Autodesk Fusion 360 part; units mm, degrees
sketch "Sketch1" plane through (0, 0, 0) normal (0, 0, 1) x (1, 0, 0)
  circle A0 centre (0, 0) radius 3.45
  circle A1 centre (0, 0) radius 4.45
  dimension "d1" = 6.9
  dimension "d2" = 1
extrude "Extrude1" add sketch "Sketch1" along normal blind 3
extrude "Extrude2" add sketch "Sketch1" along normal blind 6 contours A0
sketch "Sketch2" plane through (0, 0, 6) normal (0, 0, 1) x (-1, 0, 0)
  circle A0 centre (0, 0) radius 3.45
  circle A1 centre (-2, 2) radius 0.5
  circle A2 centre (0, 2) radius 0.5
  circle A3 centre (2, 2) radius 0.5
  circle A4 centre (-2, 0) radius 0.5
  circle A5 centre (0, 0) radius 0.5
  circle A6 centre (2, 0) radius 0.5
  circle A7 centre (-2, -2) radius 0.5
  circle A8 centre (0, -2) radius 0.5
  circle A9 centre (2, -2) radius 0.5
  point P0 (-2, 2)
  dimension "d7" = 1
  dimension "d8" = 1
  dimension "d9" = 1
  dimension "d10" = 1
  dimension "d11" = 1
  dimension "d12" = 1
  dimension "d13" = 1
  dimension "d14" = 1
  dimension "d15" = 1
hole "Hole2" at (0, 0, 6) direction (0, 0, -1) diameter 5 depth 4.5 tip angle 118
sketch "Sketch3" plane through (0, 0, 0) normal (0, 0, -1) x (1, 0, 0)
  circle A0 centre (0, 0) radius 0.0036
  circle A1 centre (0, 0) radius 4.45
  circle A2 centre (0, 0) radius 2
  dimension "d22" = 4
extrude "Extrude3" add sketch "Sketch3" along normal blind 5 contours A2
Verification items for the finished model (mm, model axes). A direction names the side the tool comes from. Give positions to 0.01 mm unless a question says otherwise; leave off trailing zeros. Loops run counter-clockwise (first coordinate to the right, second up) from the corner with the lowest first, then second, coordinate; pieces in that order, holes last.
1) Sectioned sample at B-B, the plane y = -2.75. Enter the section's corners in (x, z), then the cut area to 3 significant figures.
2) Sectioned sample at A-A, the plane z = 2.25. Enter the section's corners in (x, y), then the cut area to 3 significant figures.
3) Depth check by flat-ended pin: pin 1 Ø1.5 at (x, z) = (1.5, 4.5) entering from -Y; pin 2 Ø3 at (x, z) = (2.5, 3.5) entering from -Y; pin 3 Ø4.5 at (x, y) = (1, -0.5) entering from +Z; pin 4 Ø4 at (x, z) = (0.5, -2.5) entering from +Y. Enter the tip coordinate at first touch or a pass-through.
4) Sectioned sample at C-C, the plane z = -1.25. Enter the section's corners in (x, y).
5) Thickness scan on line 1 along Y through (x, z) = (0, 2.45); line 2 along Y through (x, z) = (0, 4.9); line 3 along X through (y, z) = (1, 3.25). Record the ranges inside material, lowest first.
6) Draft check along Y on faces 4 (the flat face through (0, 0.4, -5)), 5 (the cylindrical face through (-0.965, 4.344, 1.479)), 6 (the conical face through (-0.43, 0.09, 0.26)). Enter one of: pulls with the +Y half, pulls with the -Y half, needs draft (parallel to the pull), parting line crosses it, or undercut.
7) Set-up check for faces 1 (the flat face through (2, 2, 6)), 2 (the cylindrical face through (2.44, 0.54, 3.72)), 3 (the flat face through (2, -1, 0)): record each of +Z, -Z, +X, -X, +Y, -Y from which the full face is reachable in a straight line by a thin tool's end or side.
Answers:
1. outline: (-3.5, 0) - (3.5, 0) - (3.5, 3) - (2.08, 3) - (2.08, 6) - (-2.08, 6) - (-2.08, 3) - (-3.5, 3) - close
1. area: 33.5 mm2
2. outline: circle Ø8.9 at (0, 0); hole circle Ø5 at (0, 0)
2. area: 42.6 mm2
3. pin 1: stops at y = -3.37
3. pin 2: stops at y = -4.32
3. pin 3: stops at z = 6
3. pin 4: stops at y = 2
4. outline: circle Ø4 at (0, 0); hole circle Ø0.01 at (0, 0)
5. line 1: y = -4.45 to -2.5, 2.5 to 4.45
5. line 2: y = -3.45 to -2.5, 2.5 to 3.45
5. line 3: x = -3.3 to -2.29, 2.29 to 3.3
6. face 4: needs draft
6. face 5: parting line crosses it
6. face 6: undercut
7. face 1: +Z, +X, -X, +Y, -Y
7. face 2: +Z
7. face 3: -Z
